Can you work these out from the model? Positions are in its coordinate system, mm. Coordinates: 2 decimals unless noted, no trailing zeros. Order: outer loops, then holes, each group sorted by start corner. A loop starts at its lowest first (then second) coordinate and runs counter-clockwise, first axis right, second up. Notation, with made-up numbers: (-31, 55) - (-14, 55) arc R25 cw to (-14, 81) - close; hole circle Ø1 at (-7, 24.25). An arc over 180 degrees is marked (long way). Use a Markdown table: item, result. Add a question column.
(1) If I drill on L1, parallel to X at y = -2.9, z = 16.5; L2, parallel to X at y = -3.85, z = -11; L3, parallel to X at y = -1.85, z = 8, over which ranges is the centre line in solid material (lowest first)? Write a range as [from, to].
(2) I want a section at A-A (y = -3.8). List the corners of the cut face in (x, z) for me, and give its area (3 significant figures).
(3) For pin 1 Ø1.5 at (x, z) = (71.5, -9) entering from -Y; pin 2 Ø1.5 at (y, z) = (-4, -1.5) entering from +X, each with a flat end and sliding along its axis, tell me the tip position at first contact or that it passes through.
```python
from build123d import *

# Parameters (mm, degrees)
F0_W     = 150
F0_H     = 75
F1_DEPTH = 4.8
F2_W     = 5
F2_H     = 75
F3_DEPTH = 2
F4_R     = 1.99999


# Not quite as in the source:
# - a fillet or chamfer is up to 0.001 mm smaller than in the source, because OpenCascade refuses the exact size


with BuildPart() as f1:
    # F0 (on Front) → F1 (new body)
    with BuildSketch(Plane.XZ):
        Rectangle(F0_W, F0_H)
    extrude(amount=F1_DEPTH)

    # F2 (on face) → F3 (cut)
    with BuildSketch(Plane.XZ.offset(4.8)):
        with Locations((70.5, 0)):
            Rectangle(F2_W, F2_H)
    extrude(amount=-F3_DEPTH, mode=Mode.SUBTRACT)

    # F4 (radius 2 in the source; OpenCascade refuses exactly that, so slightly less here)
    f4_edges = [f1.edges().sort_by_distance(p)[0] for p in [
        (75, 0, 0),
        (75, -4.8, 0),
    ]]
    fillet(f4_edges, radius=F4_R)


solid = f1.part
```
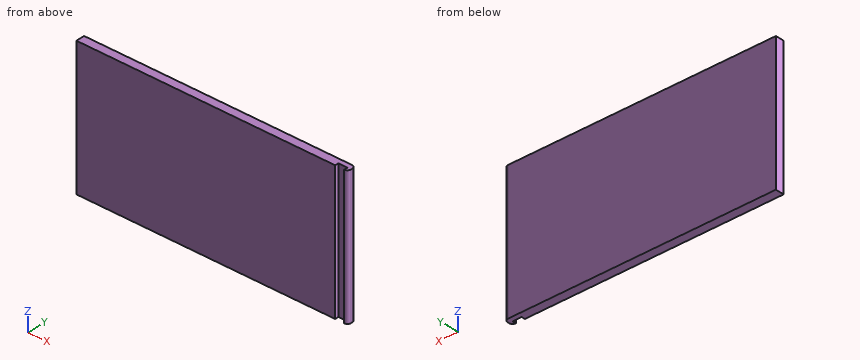
Answers follow:
| question | item | result |
|---|---|---|
| 1 | L1 | x = [-75, 68], [73, 75] |
| 1 | L2 | x = [-75, 68], [73, 74.7] |
| 1 | L3 | x = [-75, 74.99] |
| 2 | outline | (-75, -37.5) - (68, -37.5) - (68, 37.5) - (-75, 37.5) - close; (73, -37.5) - (74.73, -37.5) - (74.73, 37.5) - (73, 37.5) - close |
| 2 | area | 10,900 mm² |
| 3 | pin 1 | stops at y = -2.8 |
| 3 | pin 2 | stops at x = 74.95 |
